Autodesk Inventor part; units mm, degrees
ref_plane "YZ Plane" through (0, 0, 0) normal (1, 0, 0) x (0, 1, 0)
ref_plane "XZ Plane" through (0, 0, 0) normal (0, 1, 0) x (-1, 0, 0)
ref_plane "XY Plane" through (0, 0, 0) normal (0, 0, 1) x (1, 0, 0)
sketch "Sketch1" plane through (0, 0, 0) normal (0, 1, 0) x (-1, 0, 0)
  circle A0 centre (0, 0) radius 1.8415
  circle A1 centre (0, -42.8625) radius 1.8415
  line L0 (0, 0) -> (0, -42.8625) construction
  circle A2 centre (1.742, -13.4938) radius 3.3655
  circle A3 centre (1.742, -29.3687) radius 1.7145
  line L1 (1.742, -29.3687) -> (1.742, -13.4938) construction
  circle A4 centre (0, 0) radius 3.81
  circle A5 centre (0, -42.8625) radius 3.81
  circle A6 centre (1.742, -13.4938) radius 5.715
  circle A7 centre (1.742, -29.3687) radius 3.81
  line L2 (7.2517, -11.9756) -> (3.6731, 1.0121)
  line L3 (-3.8097, 0.0461) -> (-3.9726, -13.4247)
  line L4 (-3.9305, -14.1898) -> (-2.068, -29.3687)
  line L5 (7.4157, -14.1796) -> (5.5245, -29.826)
  line L6 (3.7786, -43.3503) -> (5.5245, -29.826)
  line L7 (-3.7775, -42.3657) -> (-2.068, -29.3687)
  point P0 (-37.12, -21.4312)
  point P1 (0, -21.4312)
  point P2 (1.742, -21.4312)
  dimension "d0" = 3.683
  dimension "d1" = 42.8625
  dimension "d2" = 42.8625
  dimension "d3" = 6.731
  dimension "d4" = 3.429
  dimension "d5" = 15.875
  dimension "d6" = 38.862
  dimension "d7" = 7.62
  dimension "d8" = 11.43
  dimension "d9" = 7.62
extrude "Extrusion1" add sketch "Sketch1" along normal blind 3.175
sketch "Sketch2" plane through (0, 3.175, 0) normal (0, 1, 0) x (1, 0, 0)
  circle A0 centre (-1.742, 13.4938) radius 3.3655
  circle A1 centre (0, 0) radius 1.8415
  circle A2 centre (-1.742, 29.3687) radius 1.7145
  circle A3 centre (0, 42.8625) radius 1.8415
  arc A4 (3.7775, 42.3657) -> (-3.7786, 43.3503) centre (0, 42.8625) ccw
  line L0 (-3.7786, 43.3503) -> (-5.5166, 29.8871)
  line L1 (-5.5245, 29.826) -> (-7.4157, 14.1796)
  arc A5 (-7.4157, 14.1796) -> (-7.2517, 11.9756) centre (-1.742, 13.4938) ccw
  line L2 (-7.2517, 11.9756) -> (-3.6731, -1.0121)
  arc A6 (-3.6731, -1.0121) -> (3.8097, -0.0461) centre (0, 0) ccw
  line L3 (3.8097, -0.0461) -> (3.9726, 13.4247)
  arc A7 (3.9726, 13.4247) -> (3.9305, 14.1898) centre (-1.742, 13.4938) ccw
  line L4 (3.9305, 14.1898) -> (2.068, 29.3687)
  line L5 (2.068, 29.3687) -> (3.7775, 42.3657)
  arc A8 (-5.5166, 29.8871) -> (-5.5245, 29.826) centre (-1.742, 29.3687) ccw
extrude "Extrusion2" add sketch "Sketch2" along normal blind 1.27 contours A0 | A2 | L5 L4 A7 L3 A6 L2 A5 L1 A8 L0 A4
fillet "Fillet1" radius 3.175 1 edges at (2.068, 2.2225, -29.3687)
properties part number "CarrageRodEndMount" material "ABS Plastic"
Geometry check sheet. Reference: the model listing, model coordinates, mm. A direction names the side the tool comes from. Give positions to 0.01 mm unless a question says otherwise; leave off trailing zeros. Write each loop counter-clockwise with the first axis right and the second up, starting at its lowest first coordinate (ties: lowest second). Pieces come first, ordered by that corner, then holes. Notation, with made-up numbers: (13, -13.5) -> (48, -13.5) arc R24 cw to (48, 23.5) -> close; hole circle Ø11 at (-24, 24). An arc over 180 degrees is marked (long way). One line per question, with ' | ' between items.
Item 1: Depth check by flat-ended pin: pin 1 (1.5 mm diameter, centred on y = 2.5, z = -22.5, fed in from -X); pin 2 (3 mm diameter, centred on x = -1.74, z = -29.37, fed in from -Y) (3 decimals); pin 3 (3 mm diameter, centred on x = 0, z = 0, fed in from +Y); pin 4 (1.5 mm diameter, centred on x = -2.5, y = 2, fed in from -Z). Enter the tip coordinate at first touch or a pass-through.
Determined:
pin 1: x = -6.5 | pin 2: y = 3.175 | pin 3: through | pin 4: z = -46.25
Item 2: Sectioned sample at B-B, the plane z = -15. Record the boundary of the cut face in (x, y) (3 decimals), plus the area to 3 significant figures.
Determined:
outline: (-7.317, 0) -> (-4.752, 0) -> (-4.752, 3.175) -> (1.268, 3.175) -> (1.268, 0) -> (3.831, 0) -> (3.831, 4.445) -> (-7.317, 4.445) -> close | area: 30.4 mm^2
Item 3: Scan lines: line 1 along Z through (x, y) = (-0.75, 2.4); line 2 along Z through (x, y) = (-3, 2.75); line 3 along Y through (x, z) = (-0.75, -30.5) (3 decimals). Record each from-to range of solid material in increasing order.
Determined:
line 1: -46.6 to -44.54, -41.18 to -30.77, -27.97 to -16.71, -10.28 to -1.68, 1.68 to 3.74 | line 2: -45.21 to -30.53, -28.2 to -16.62, -10.37 to 2.35 | line 3: 3.175 to 4.445
Item 4: Draft check along Z on faces 1 (the flat face through (-6.483, 2.191, -21.893)), 2 (the flat face through (3.037, 2.191, -21.476)), 3 (the flat face through (-1, 4.445, -22)). Enter one of: released by +Z, released by -Z, zero draft, split by the parting line, or undercut.
Determined:
face 1: released by -Z | face 2: undercut | face 3: zero draft
Item 5: Access from +Z, -Z, +X, -X, +Y, -Y to the whole of each face (thin tool, end or side, straight path). Record for faces 4 (the flat face through (2.96, 2.19, -36.16)), 5 (the flat face through (0, 0, -21)), 6 (the flat face through (-2, 3.175, -14)).
Determined:
face 4: +X, +Y, -Y | face 5: +Z, -Z, +X, -X, -Y | face 6: -Y
Item 6: Sectioned sample at A-A, the plane y = 1.9. State how many separate pieces and enclosed holes the cut face has, plus the area to 3 significant figures.
Determined:
separate pieces: 1 | enclosed holes: 4 | area: 366 mm^2
Item 7: Sectioned sample at D-D, the plane z = -7. Record the boundary of the cut face in (x, y) (3 decimals).
Determined:
outline: (-5.881, 0) -> (3.895, 0) -> (3.895, 4.445) -> (-5.881, 4.445) -> close
